```python
from build123d import *

# Parameters (mm, degrees)
F0_R     = 9.5
F1_DEPTH = 82
F2_R     = 2.5
F3_DEPTH = 25
F6_R     = 2
F7_DEPTH = 5


with BuildPart() as f1:
    # F0 (on Front) → F1 (new body)
    with BuildSketch(Plane.XZ):
        with BuildLine():
            ThreePointArc((10.8166538264, -2), (10.9540675571, -1.004193186), (11, 0))
            ThreePointArc((11, 0), (10.9540675571, 1.004193186), (10.8166538264, 2))
            ThreePointArc((10.8166538264, 2), (-11, 0), (10.8166538264, -2))
        make_face()
        Circle(F0_R, mode=Mode.SUBTRACT)
        with BuildLine():
            ThreePointArc((10.8166538264, 2), (10.9540675571, 1.004193186), (11, 0))
            ThreePointArc((11, 0), (10.9540675571, -1.004193186), (10.8166538264, -2))
            Line((10.8166538264, -2), (26, -2))
            Line((26, -2), (26, 2))
            Line((26, 2), (10.8166538264, 2))
        make_face()
    extrude(amount=-F1_DEPTH)

    # F2 (on face) → F3 (cut)
    with BuildSketch(Plane.XY.offset(2)):
        with Locations((18.4083269132, 72)):
            Circle(F2_R)
        with Locations((18.4083269132, 41)):
            Circle(F2_R)
        with Locations((18.4083269132, 10)):
            Circle(F2_R)
    extrude(amount=-F3_DEPTH, mode=Mode.SUBTRACT)

    # F6 (on face) → F7 (cut)
    with BuildSketch(Plane(origin=(6.6010824652, 0, 8.799188047), x_dir=(0.7999261861, 0, -0.6000984059), z_dir=(0.6000984059, 0, 0.7999261861))):
        with Locations((0, 4)):
            Circle(F6_R)
    extrude(amount=-F7_DEPTH, mode=Mode.SUBTRACT)


solid = f1.part
```
Could you check a few things on this model? Use its own coordinates, in mm. A direction names the side the tool comes from. Round coordinates to 2 decimals unless told otherwise and drop trailing zeros. Loops run counter-clockwise (first coordinate to the right, second up) from the corner with the lowest first, then second, coordinate; pieces in that order, holes last.
Q1. For P1, Ø3, axis at y = 51, z = -2, coming from the -X side; P2, Ø12, axis at x = 17.5, y = 50, coming from the -Z side; P3, Ø8, axis at x = 18.41, y = 10, coming from the +Z side; P4, Ø4, axis at x = 18.41, y = 41, coming from the -Z side, each with a flat end and sliding along its axis, tell me the tip position at first contact or that it passes through.
Q2. On a 3-axis mill with a long thin cutter (end or side, diameter ignored), from which of +Z, -Z, +X, -X, +Y, -Y can I reach the whole of each face in a straight line? I mean faces 4 (the cylindrical face through (19.56, 7.78, 0.03)), 5 (the flat face through (22, 40, -2)). Say none if no direction works.
Q3. Thinking about a two-plate mould opening in Z: for faces 1 (the flat face through (15, 40, 2)), 2 (the cylindrical face through (4.82, 2.78, 9.07)), 3 (the flat face through (10, 0, 1)), which applies, pulls with the +Z half, pulls with the -Z half, needs draft (parallel to the pull), parting line crosses it, or undercut?
Q4. I want a section at D-D (z = 4.25). Write out the boundary of the cut face in (x, y), and give its area (3 significant figures).
Q5. I want a section at A-A (y = 72). Write out the boundary of the cut face in (x, z).
Q6. Please list where these lines run through material, in increasing order: L1, parallel to Z at x = 0.5, y = 22.5; L2, parallel to Z at x = 24, y = 35; L3, parallel to Z at x = -8, y = 25.5.
Q7. I want a section at C-C (x = 0). Write out the boundary of the cut face in (y, z).
Q8. I want a section at B-B (z = 0). Write out the boundary of the cut face in (x, y), and give its area (3 significant figures).
Answer below:
1. P1: stops at x = -10.99
1. P2: stops at z = -2
1. P3: stops at z = 2
1. P4: passes through
2. face 4: +Z, -Z
2. face 5: -Z, +X, +Y, -Y
3. face 1: pulls with the +Z half
3. face 2: undercut
3. face 3: needs draft
4. outline: (-10.15, 0) - (-8.5, 0) - (-8.5, 82) - (-10.15, 82) - close; (8.5, 0) - (10.15, 0) - (10.15, 82) - (8.5, 82) - close
4. area: 271 mm2
5. outline: (10.82, -2) - (15.91, -2) - (15.91, 2) - (10.82, 2) arc R11 ccw (long way) to start; (20.91, -2) - (26, -2) - (26, 2) - (20.91, 2) - close; hole circle Ø19 at (0, 0)
6. L1: z = -10.99 to -9.49, 9.49 to 10.99
6. L2: z = -2 to 2
6. L3: z = -7.55 to -5.12, 5.12 to 7.55
7. outline: (0, -11) - (82, -11) - (82, -9.5) - (0, -9.5) - close; (0, 9.5) - (82, 9.5) - (82, 11) - (0, 11) - close
8. outline: (-11, 0) - (-9.5, 0) - (-9.5, 82) - (-11, 82) - close; (9.5, 0) - (26, 0) - (26, 82) - (9.5, 82) - close; hole circle Ø5 at (18.41, 10); hole circle Ø5 at (18.41, 41); hole circle Ø5 at (18.41, 72)
8. area: 1,420 mm2
